Geometry check sheet. Reference: drawing and pictorial views, mm from the part's lowest x, y, z. A direction names the side the tool comes from. Round coordinates to 2 decimals unless told otherwise and drop trailing zeros. Loops run counter-clockwise (first coordinate to the right, second up) from the corner with the lowest first, then second, coordinate; pieces in that order, holes last. Notation, with made-up numbers: (70.5, 10) -> (112.5, 10) arc R29 ccw to (112.5, 49) -> close; hole circle Ø1 at (-34, 49). An arc over 180 degrees is marked (long way). Write item = value, one per line.
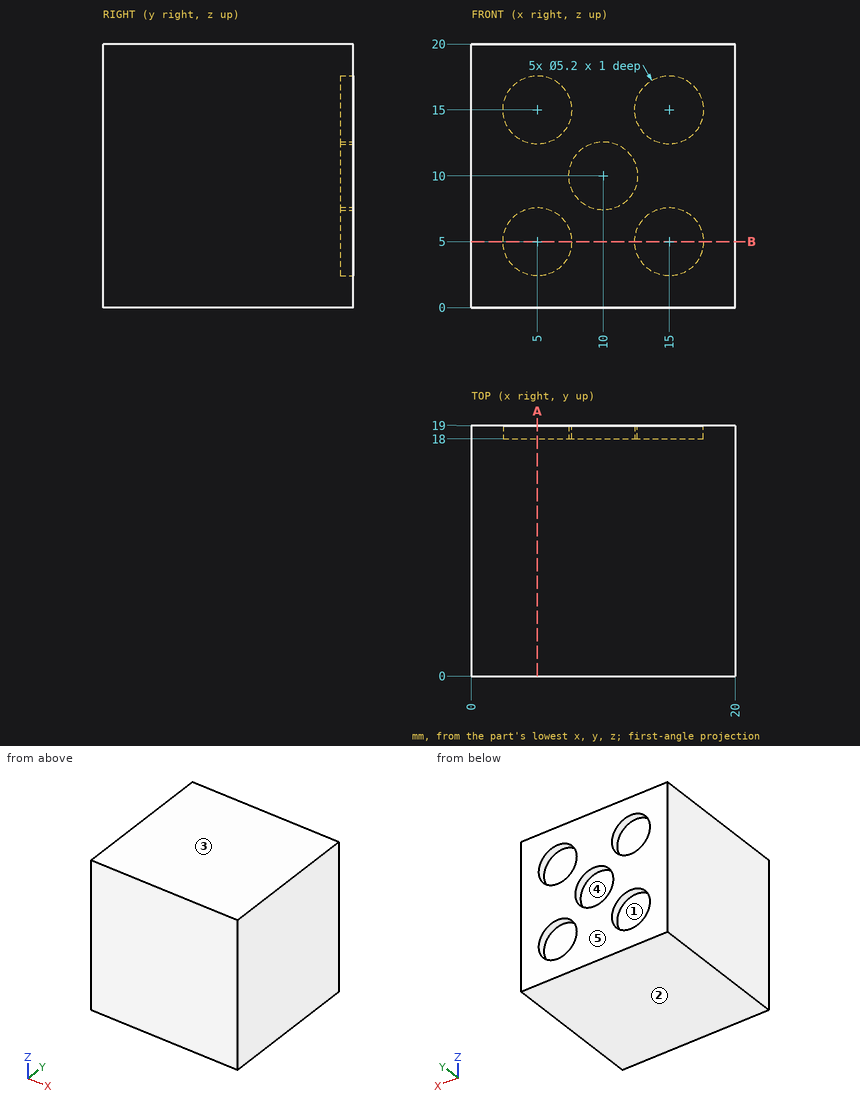
(1) Sectioned sample at A-A, the plane x = 5. Record the cut outline in (y, z), and give its area (3 significant figures).
Filled sheet:
outline = (0, 0) -> (19, 0) -> (19, 2.4) -> (18, 2.4) -> (18, 7.6) -> (19, 7.6) -> (19, 12.4) -> (18, 12.4) -> (18, 17.6) -> (19, 17.6) -> (19, 20) -> (0, 20) -> close
area = 370 mm2
(2) Sectioned sample at B-B, the plane z = 5. Record the cut outline in (x, y).
Filled sheet:
outline = (0, 0) -> (20, 0) -> (20, 19) -> (17.6, 19) -> (17.6, 18) -> (12.4, 18) -> (12.4, 19) -> (7.6, 19) -> (7.6, 18) -> (2.4, 18) -> (2.4, 19) -> (0, 19) -> close
(3) Draft check along Z on the marked faces 3, 4 and 5. Enter one of: released by +Z, released by -Z, zero draft, split by the parting line, or undercut.
Filled sheet:
face_3 = released by +Z
face_4 = undercut
face_5 = zero draft
(4) Go/stop test with flat-tipped pins: pin 1 Ø8 at (y, z) = (4.5, 5) entering from -X; pin 2 Ø1.6 at (x, z) = (11, 10.5) entering from +Y. Record where each tip stops, or that it passes through.
Filled sheet:
pin_1 = 0
pin_2 = 18
(5) Set-up check for the marked faces 1 and 2: record each of +Z, -Z, +X, -X, +Y, -Y from which the full face is reachable in a straight line by a thin tool's end or side.
Filled sheet:
face_1 = +Y
face_2 = -Z, +X, -X, +Y, -Y
(6) Material ranges on probe 1 along Z at (x, y) = (15, 18.45); probe 2 along Z at (x, y) = (10, 18.4); probe 3 along Y at (x, z) = (13.75, 5), recorded low to high. Write a range as from..to.
Filled sheet:
probe_1 = 0..2.4, 7.6..12.4, 17.6..20
probe_2 = 0..7.4, 12.6..20
probe_3 = 0..18
